Model file for the job. Use its own axes, mm. Face numbers are marked on the shaded views. A direction names the side the tool comes from. Give positions to 0.01 mm unless a question says otherwise; leave off trailing zeros. Loops run counter-clockwise (first coordinate to the right, second up) from the corner with the lowest first, then second, coordinate; pieces in that order, holes last. Notation, with made-up numbers: M 29,-4 L 34,-4 A18 ccw 34,31 Z; hole C 88.5,-15 d5. An arc over 180 degrees is marked long. Use CSV: the item, a comma, the result in double quotes. Start each with the question number.
(1) Flat gauge pins, fed straight in: P1, Ø9, axis at x = 23.55, y = 23.55, coming from the -Z side; P2, Ø3, axis at x = 45.5, y = 15.5, coming from the +Z side; P3, Ø4.5, axis at x = -23.55, y = -23.55, coming from the +Z side; P4, Ø4.5, axis at x = -45, y = -19.5, coming from the +Z side. Where does each tip first touch, or does it go through?
(2) Wall check: line 1 along Y through (x, z) = (-23, -3); line 2 along Y through (x, z) = (23.55, -7.25); line 3 along X through (y, z) = (41, 0). Give the ranges that are in metal, low to high. Write a range as from..to.
(3) Slice it at C-C on z = -40. List the corners of the cut face in (x, y) (3 decimals), and give its area (3 significant figures).
(4) Slice it at D-D on y = 15.7. List the corners of the cut face in (x, z), and give its area (3 significant figures).
(5) Tool access for the marked faces 4, 5 and 6: list every direction of +Z, -Z, +X, -X, +Y, -Y with a clear straight run to the whole face (end or side of a thin tool).
(6) Two-plate mould, pull along X, no slides. Class the marked faces 1, 2 and 3: pulls with the +X half, pulls with the -X half, needs draft (parallel to the pull), parting line crosses it, or undercut.
(7) Slice it at A-A on x = 57. List the corners of the cut face in (y, z), and give its area (3 significant figures).
(8) Slice it at B-B on y = -30. List the corners of the cut face in (x, z).
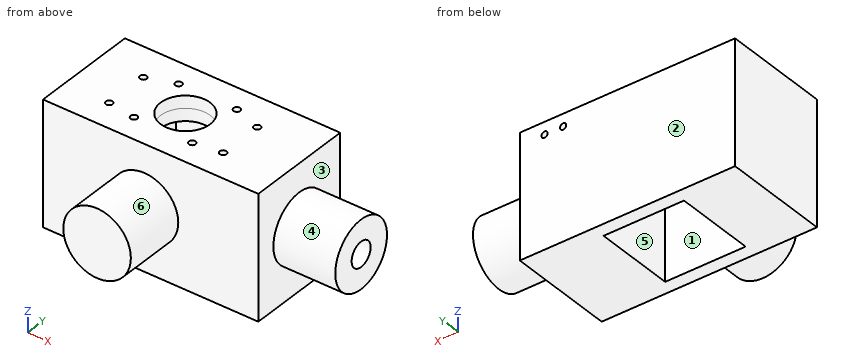
Autodesk Inventor part; units mm, degrees
ref_plane "YZ Plane" through (0, 0, 0) normal (1, 0, 0) x (0, 1, 0)
ref_plane "XZ Plane" through (0, 0, 0) normal (0, 1, 0) x (-1, 0, 0)
ref_plane "XY Plane" through (0, 0, 0) normal (0, 0, 1) x (1, 0, 0)
sketch "Sketch1" plane through (0, 0, 0) normal (0, 0, 1) x (1, 0, 0)
  line L0 (-23.55, 23.55) -> (23.55, 23.55) construction
  line L1 (23.55, 23.55) -> (23.55, -23.55) construction
  line L2 (23.55, -23.55) -> (-23.55, -23.55) construction
  line L3 (-23.55, -23.55) -> (-23.55, 23.55) construction
  line L4 (0, 23.55) -> (0, -23.55) construction
  line L5 (-23.55, 0) -> (23.55, 0) construction
  circle A0 centre (-23.55, 23.55) radius 2.75
  circle A1 centre (23.55, 23.55) radius 2.75
  circle A2 centre (-23.55, -23.55) radius 2.75
  circle A3 centre (23.55, -23.55) radius 2.75
  circle A4 centre (0, 0) radius 20
  line L6 (-28.2, 28.2) -> (28.2, 28.2) construction
  line L7 (28.2, 28.2) -> (28.2, -28.2) construction
  line L8 (28.2, -28.2) -> (-28.2, -28.2) construction
  line L9 (-28.2, -28.2) -> (-28.2, 28.2) construction
  line L10 (-28.2, 0) -> (28.2, 0) construction
  line L11 (0, -28.2) -> (0, 28.2) construction
  line L12 (-60, 21.2) -> (-32, 21.2) construction
  line L13 (-32, 21.2) -> (-32, -25.8) construction
  line L14 (-32, -25.8) -> (-60, -25.8) construction
  line L15 (-60, -25.8) -> (-60, 21.2) construction
  line L16 (-46, 21.2) -> (-46, -25.8) construction
  line L17 (-60, -2.3) -> (-32, -2.3) construction
  circle A5 centre (-46, 15.7) radius 2.75
  circle A6 centre (-46, -20.3) radius 2.75
  line L18 (60, 21.2) -> (32, 21.2) construction
  line L19 (32, 21.2) -> (32, -25.8) construction
  line L20 (32, -25.8) -> (60, -25.8) construction
  line L21 (60, -25.8) -> (60, 21.2) construction
  line L22 (46, 21.2) -> (46, -25.8) construction
  line L23 (60, -2.3) -> (32, -2.3) construction
  circle A7 centre (46, 15.7) radius 2.75
  circle A8 centre (46, -20.3) radius 2.75
  line L24 (-82, 43.2) -> (82, 43.2)
  line L25 (82, 43.2) -> (82, -43.2)
  line L26 (82, -43.2) -> (-82, -43.2)
  line L27 (-82, -43.2) -> (-82, 43.2)
  point P0 (0, 0)
  dimension "d0" = 47.1
  dimension "d1" = 47.1
  dimension "d2" = 5.5
  dimension "d4" = 40
  dimension "d5" = 56.4
  dimension "d6" = 56.4
  dimension "d9" = 46
  dimension "d10" = 47
  dimension "d11" = 28
  dimension "d12" = 5.5
  dimension "d13" = 36
  dimension "d14" = 22
  dimension "d15" = 15
  dimension "d18" = 2.3
extrude "Extrusion1" add sketch "Sketch1" along normal blind 10
sketch "Sketch2" plane through (0, 0, 0) normal (0, 0, -1) x (-1, 0, 0)
  line L0 (32.5, -32.5) -> (-32.5, -32.5)
  line L1 (-32.5, -32.5) -> (-32.5, 32.5)
  line L2 (-32.5, 32.5) -> (32.5, 32.5)
  line L3 (32.5, 32.5) -> (32.5, -32.5)
  line L4 (0, 32.5) -> (0, -32.5) construction
  line L5 (-32.5, 0) -> (32.5, 0) construction
  line L6 (-82, -43.2) -> (-82, 43.2)
  line L7 (82, -43.2) -> (-82, -43.2)
  line L8 (-82, 43.2) -> (82, 43.2)
  line L9 (82, 43.2) -> (82, -43.2)
  line L10 (82, -43.2) -> (-82, -43.2)
  line L11 (-82, -43.2) -> (-82, 43.2)
  point P0 (0, 0)
  point P1 (0, 0)
  dimension "d19" = 65
  dimension "d20" = 65
extrude "Extrusion2" add sketch "Sketch2" along normal blind 90
sketch "Sketch3" plane through (0, 0, 0) normal (0, 0, -1) x (-1, 0, 0)
  line L0 (32.5, -32.5) -> (32.5, 32.5)
  line L1 (32.5, 32.5) -> (-32.5, 32.5)
  line L2 (-32.5, 32.5) -> (-32.5, -32.5)
  line L3 (-32.5, -32.5) -> (32.5, -32.5)
  circle A0 centre (23.55, 23.55) radius 2.75
  circle A1 centre (-23.55, 23.55) radius 2.75
  circle A2 centre (23.55, -23.55) radius 2.75
  circle A3 centre (-23.55, -23.55) radius 2.75
  circle A4 centre (0, 0) radius 20
extrude "Extrusion3" add sketch "Sketch3" along normal blind 10
sketch "Sketch8" plane through (82, -43.2, 10) normal (1, 0, 0) x (0, 0, -1)
  line L0 (100, 86.4) -> (0, 86.4)
  line L1 (0, 0) -> (0, 86.4)
  line L2 (100, 0) -> (0, 0)
  line L3 (100, 86.4) -> (100, 0)
  point P0 (10, 43.2)
extrude "Extrusion8" add sketch "Sketch8" along normal blind 10
sketch "Sketch9" plane through (92, -43.2, 10) normal (1, 0, 0) x (0, 0, -1)
  line L0 (100, 86.4) -> (0, 86.4) construction
  line L1 (50, 86.4) -> (50, 0) construction
  line L2 (0, 0) -> (100, 0) construction
  line L3 (100, 75.7) -> (100, 10.7) construction
  line L4 (100, 43.2) -> (0, 43.2) construction
  line L5 (0, 23.2) -> (0, 63.2) construction
  circle A0 centre (50, 43.2) radius 27.305
  point P0 (10, 43.2)
  dimension "d38" = 54.61
extrude "Extrusion9" add sketch "Sketch9" along normal blind 50
sketch "Sketch10" plane through (-82, -43.2, -90) normal (0, -1, 0) x (1, 0, 0)
  line L0 (0, 0) -> (0, 100) construction
  line L1 (0, 50) -> (174, 50) construction
  line L2 (174, 100) -> (174, 0) construction
  line L3 (62, 100) -> (102, 100) construction
  line L4 (82, 100) -> (82, 0) construction
  line L5 (49.5, 0) -> (114.5, 0) construction
  circle A0 centre (82, 50) radius 27.305
  point P0 (82, 90)
  dimension "d41" = 54.61
extrude "Extrusion10" add sketch "Sketch10" along normal blind 50
sketch "Sketch11" plane through (142, 0, -40) normal (1, 0, 0) x (0, 0, -1)
  circle A0 centre (0, 0) radius 27.305 construction
  circle A1 centre (0, 0) radius 10
  point P0 (-40, 0)
  dimension "d44" = 20
extrude "Extrusion11" cut sketch "Sketch11" against normal up to surface (109.5 mm away)
sketch "Sketch12" plane through (-82, 43.2, 10) normal (0, 1, 0) x (1, 0, 0)
  line L0 (174, 100) -> (174, 0) construction
  line L1 (174, 0) -> (154, 0) construction
  line L2 (154, 0) -> (154, 10) construction
  line L3 (154, 10) -> (174, 10) construction
  line L4 (174, 10) -> (174, 0) construction
  line L5 (154, 10) -> (139, 10) construction
  line L6 (139, 10) -> (139, 0) construction
  line L7 (0, 0) -> (174, 0) construction
  circle A0 centre (154, 10) radius 2.5
  circle A1 centre (139, 10) radius 2.5
  point P0 (82, 10)
  dimension "d47" = 20
  dimension "d48" = 10
  dimension "d49" = 15
  dimension "d50" = 5
  dimension "d51" = 5
extrude "Extrusion12" cut sketch "Sketch12" against normal blind 6
properties part number "driver_L"
Reply:
1,P1,"stops at z = -10"
1,P2,"stops at z = 0"
1,P3,"passes through"
1,P4,"stops at z = 10"
2,line 1,"y = -43.2..-26.24, -20.86..20.86, 26.24..43.2"
2,line 2,"y = -43.2..-26.3, -20.8..20.8, 26.3..43.2"
2,line 3,"x = -82..54.5, 59.5..69.5, 74.5..92"
3,outline,"M -82,-43.2 L -27.305,-43.2 L -27.305,-93.2 L 27.305,-93.2 L 27.305,-43.2 L 92,-43.2 L 92,-27.305 L 142,-27.305 L 142,-10 L 32.5,-10 L 32.5,-32.5 L -32.5,-32.5 L -32.5,32.5 L 32.5,32.5 L 32.5,10 L 142,10 L 142,27.305 L 92,27.305 L 92,43.2 L -82,43.2 Z"
3,area,"14,100 mm^2"
4,outline,"M -82,-90 L -32.5,-90 L -32.5,-10 L -12.39,-10 L -12.39,10 L -43.25,10 L -43.25,0 L -48.75,0 L -48.75,10 L -82,10 Z; M 12.39,-10 L 32.5,-10 L 32.5,-90 L 92,-90 L 92,-62.34 L 142,-62.34 L 142,-17.66 L 92,-17.66 L 92,10 L 48.75,10 L 48.75,0 L 43.25,0 L 43.25,10 L 12.39,10 Z"
4,area,"13,800 mm^2"
5,face 4,"+X"
5,face 5,"-Z"
5,face 6,"-Y"
6,face 1,"undercut"
6,face 2,"needs draft"
6,face 3,"pulls with the +X half"
7,outline,"M -43.2,-90 L 43.2,-90 L 43.2,-2.5 L 37.2,-2.5 L 37.2,2.5 L 43.2,2.5 L 43.2,10 L -43.2,10 Z; hole C 0,-40 d20"
7,area,"8,300 mm^2"
8,outline,"M -82,-90 L -32.5,-90 L -32.5,-10 L 32.5,-10 L 32.5,-90 L 92,-90 L 92,10 L -82,10 Z"
